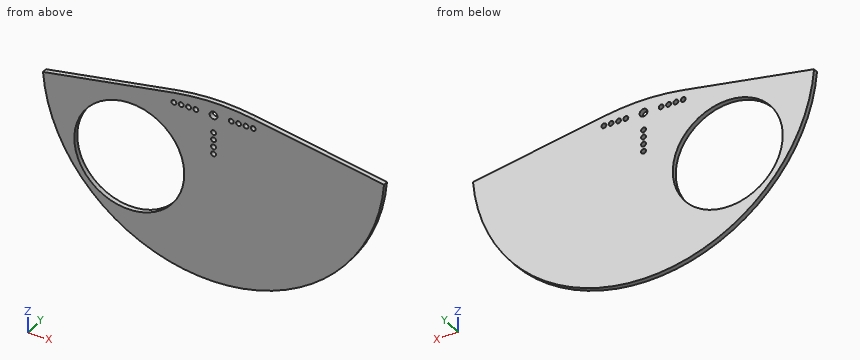
from build123d import *

# Parameters (mm, degrees)
SKETCH_1_R      = 1
SKETCH_1_R_2    = 1.6
SKETCH_1_R_3    = 22.5
EXTRUDE_1_DEPTH = 1


with BuildPart() as part:
    # 草圖1 → 填料-伸長1 (new, symmetric)
    with BuildSketch(Plane(origin=(0, 0, 0), x_dir=(1, 0, 0), z_dir=(0, 1, 0))):
        with BuildLine():
            Line((-69.788277988, 5.440244057), (-16.249993495, -4))
            ThreePointArc((-16.249993495, -4), (0, -5.421690213), (16.249993495, -4))
            Line((16.249993495, -4), (69.788277988, 5.440244057))
            ThreePointArc((69.788277988, 5.440244057), (0, 70), (-69.788277988, 5.440244057))
        make_face()
        with Locations(Location((16.249993495, 0, 0), (0, 0, 270))):
            Circle(SKETCH_1_R, mode=Mode.SUBTRACT)
        with Locations(Location((13.249989391, 0, 0), (0, 0, 270))):
            Circle(SKETCH_1_R, mode=Mode.SUBTRACT)
        with Locations(Location((10.249991793, 0, 0), (0, 0, 270))):
            Circle(SKETCH_1_R, mode=Mode.SUBTRACT)
        with Locations(Location((7.249994195, 0, 0), (0, 0, 270))):
            Circle(SKETCH_1_R, mode=Mode.SUBTRACT)
        with Locations(Location((-16.249993495, 0, 0), (0, 0, 270))):
            Circle(SKETCH_1_R, mode=Mode.SUBTRACT)
        with Locations(Location((-13.249989391, 0, 0), (0, 0, 270))):
            Circle(SKETCH_1_R, mode=Mode.SUBTRACT)
        with Locations(Location((-10.249991793, 0, 0), (0, 0, 270))):
            Circle(SKETCH_1_R, mode=Mode.SUBTRACT)
        with Locations(Location((-7.249994195, 0, 0), (0, 0, 270))):
            Circle(SKETCH_1_R, mode=Mode.SUBTRACT)
        with Locations(Location((0, 16.249993495, 0), (0, 0, 270))):
            Circle(SKETCH_1_R, mode=Mode.SUBTRACT)
        with Locations(Location((0, 13.249989391, 0), (0, 0, 270))):
            Circle(SKETCH_1_R, mode=Mode.SUBTRACT)
        with Locations(Location((0, 10.249991793, 0), (0, 0, 270))):
            Circle(SKETCH_1_R, mode=Mode.SUBTRACT)
        with Locations(Location((0, 7.249994195, 0), (0, 0, 270))):
            Circle(SKETCH_1_R, mode=Mode.SUBTRACT)
        with Locations(Location((0, 0, 0), (0, 0, 270))):
            Circle(SKETCH_1_R_2, mode=Mode.SUBTRACT)
        with Locations(Location((-34.47199994, 28.925442436, 0), (0, 0, 270))):
            Circle(SKETCH_1_R_3, mode=Mode.SUBTRACT)
    extrude(amount=EXTRUDE_1_DEPTH, both=True)


solid = part.part
For this review, take the finished solid that the model builds, in its own axes (mm). Round coordinates to 2 decimals unless told otherwise and drop trailing zeros. Order: outer loops, then holes, each group sorted by start corner. A loop starts at its lowest first (then second) coordinate and runs counter-clockwise, first axis right, second up. Notation, with made-up numbers: (21, 62) -> (30, 62) arc R6 cw to (30, 68) -> close; hole circle Ø5 at (-36.5, 19). An arc over 180 degrees is marked (long way). Put each result on its own line as item: value.
Q1. For probe 1 along X at (y, z) = (0.35, -10); probe 2 along Z at (x, y) = (-49, -0.9); probe 3 along Z at (x, y) = (-43, -0.8), list the stretches that pass through material, from the lowest coordinate up. Write a range as [from, to].
Check result:
probe 1: [-69.28, -46.64], [-22.3, -0.97], [0.97, 69.28]
probe 2: [-49.99, -46.11], [-11.74, -1.77]
probe 3: [-55.24, -49.75], [-8.1, -0.72]
Q2. Insertion check: pin 1 Ø1.9 at (x, z) = (0, 0) entering from +Y; pin 2 Ø10 at (x, z) = (41, -60) entering from +Y. Each pin has a flat end and moves straight along its axis. Give the tip position at first contact, or say it passes through.
Check result:
pin 1: through
pin 2: y = 1
Q3. Add section C-C on y = -0.2. State how many separate pieces and enclosed holes the cut face has, plus the area to 3 significant figures.
Check result:
separate pieces: 1
enclosed holes: 14
area: 6,140 mm2
Q4. Add section B-B on z = -19.5. Write out the cut boundary in (x, y).
Check result:
outline: (-67.23, -1) -> (-54.9, -1) -> (-54.9, 1) -> (-67.23, 1) -> close; (-14.04, -1) -> (67.23, -1) -> (67.23, 1) -> (-14.04, 1) -> close
Q5. Add section D-D on x = 56.5. Write out the cut boundary in (y, z), plus the area to 3 significant figures.
Check result:
outline: (-1, -41.32) -> (1, -41.32) -> (1, -3.1) -> (-1, -3.1) -> close
area: 76.5 mm2
Q6. Add section A-A on x = -26. Write out the cut boundary in (y, z).
Check result:
outline: (-1, -64.99) -> (1, -64.99) -> (1, -49.77) -> (-1, -49.77) -> close; (-1, -8.08) -> (1, -8.08) -> (1, 2.28) -> (-1, 2.28) -> close
